Design review of the part built by this model. Coordinates are the model's own, in mm. Face numbers are marked on the shaded views. Coordinates: 2 decimals unless noted, no trailing zeros. Loops run counter-clockwise (first coordinate to the right, second up) from the corner with the lowest first, then second, coordinate; pieces in that order, holes last. Notation, with made-up numbers: (73, 87) - (94, 87) arc R16 cw to (94, 113) - close; hole circle Ø11 at (-4.75, -22). An arc over 180 degrees is marked (long way). One line per question, with ' | ' between items.
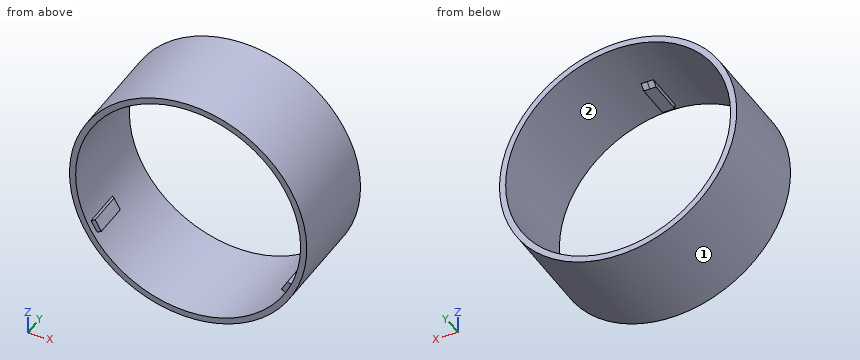
from build123d import *

# Parameters (mm, degrees)
SKETCH_1_R               = 38.5
SKETCH_1_R_2             = 36.5
EXTRUDE_1_DEPTH          = 40
EXTRUDE_3_DEPTH          = 1.6
PATTERN_CIRCULAR_1_COUNT = 3
SKETCH_3_R               = 52.927820275
CUT_EXTRUDE_1_DEPTH      = 7
CHAMFER_1_SIZE           = 1.7


with BuildPart() as part:
    # Эскиз1 → Бобышка-Вытянуть1 (new body)
    with BuildSketch(Plane(origin=(0, 0, 0), x_dir=(1, 0, 0), z_dir=(0, 1, 0))):
        with Locations(Location((0, 0, 0), (0, 0, 270))):
            Circle(SKETCH_1_R)
        with Locations(Location((0, 0, 0), (0, 0, 270))):
            Circle(SKETCH_1_R_2, mode=Mode.SUBTRACT)
    extrude(amount=EXTRUDE_1_DEPTH)

    # Эскиз2 → Бобышка-Вытянуть3 (add)
    with BuildSketch(Plane.XY.offset(36.5)):
        Polygon((1.95, 20.447072268), (-0.95, 20.447072268), (-2.05, 20.447072268), (-2.05, 9), (1.95, 9), align=None)
    extrude_3 = extrude(amount=-EXTRUDE_3_DEPTH)

    # Круговой массив1: Бобышка-Вытянуть3 ×3 about axis
    pattern_circular_1_axis = Axis((0, 0, 0), (0, 1, 0))
    for i in range(1, PATTERN_CIRCULAR_1_COUNT):
        add(extrude_3.rotate(pattern_circular_1_axis, i * 360 / PATTERN_CIRCULAR_1_COUNT))

    # Эскиз3 → Вырез-Вытянуть1 (cut)
    with BuildSketch(Plane.XZ):
        Circle(SKETCH_3_R)
    extrude(amount=-CUT_EXTRUDE_1_DEPTH, mode=Mode.SUBTRACT)

    # Фаска1
    # the kernel refuses this chamfer: 1.7 mm, written as the material it adds along each edge
    with BuildSketch(Plane(origin=(0, 20.447072268, 0), x_dir=(0, 0, 1), z_dir=(1, 0, 0))) as chamfer_1_piece_1_section:
        Polygon((36.5, -CHAMFER_1_SIZE), (36.5 - CHAMFER_1_SIZE, 0), (36.5, 0), align=None)
    chamfer_1_piece_1 = revolve(axis=Axis((0, 20.447072268, 0), (0, -1, 0)), revolution_arc=10.082397384, mode=Mode.PRIVATE)
    chamfer_1_piece_1 = split(chamfer_1_piece_1, bisect_by=Plane(origin=(-2.05, 21.014554038, 35.932884204), z_dir=(1, 0, 0)), keep=Keep.TOP, mode=Mode.PRIVATE)
    chamfer_1_piece_1 = split(chamfer_1_piece_1, bisect_by=Plane(origin=(-1.024016217, 21.014554038, 34.9), z_dir=(0, 0, 1)), keep=Keep.TOP, mode=Mode.PRIVATE)
    add(chamfer_1_piece_1)
    with BuildSketch(Plane(origin=(0, 20.447072268, 0), x_dir=(-0.9392452885856895, 0, -0.3432466866112253), z_dir=(-0.3432466866112253, 0, 0.9392452885856895))) as chamfer_1_piece_2_section:
        Polygon((36.5, -CHAMFER_1_SIZE), (36.5 - CHAMFER_1_SIZE, 0), (36.5, 0), align=None)
    chamfer_1_piece_2 = revolve(axis=Axis((0, 20.447072268, 0), (0, -1, 0)), revolution_arc=20.007603595, mode=Mode.PRIVATE)
    chamfer_1_piece_2 = split(chamfer_1_piece_2, bisect_by=Plane(origin=(-32.094466273, 21.014490137, -16.278082692), z_dir=(0.5000000000000004, 0, -0.8660254037844384)), keep=Keep.TOP, mode=Mode.PRIVATE)
    chamfer_1_piece_2 = split(chamfer_1_piece_2, bisect_by=Plane(origin=(-30.094466273, 21.014490137, -19.742184307), z_dir=(-0.5000000000000004, 0, 0.8660254037844384)), keep=Keep.TOP, mode=Mode.PRIVATE)
    chamfer_1_piece_2 = split(chamfer_1_piece_2, bisect_by=Plane(origin=(-30.199383778, 21.014490137, -17.493132939), z_dir=(-0.8660254037844384, 0, -0.5000000000000004)), keep=Keep.TOP, mode=Mode.PRIVATE)
    add(chamfer_1_piece_2)
    with BuildSketch(Plane(origin=(0, 20.447072268, 0), x_dir=(0.7668829946630015, 0, -0.6417869369944413), z_dir=(-0.6417869369944413, 0, -0.7668829946630015))) as chamfer_1_piece_3_section:
        Polygon((36.5, -CHAMFER_1_SIZE), (36.5 - CHAMFER_1_SIZE, 0), (36.5, 0), align=None)
    chamfer_1_piece_3 = revolve(axis=Axis((0, 20.447072268, 0), (0, -1, 0)), revolution_arc=20.007603595, mode=Mode.PRIVATE)
    chamfer_1_piece_3 = split(chamfer_1_piece_3, bisect_by=Plane(origin=(30.144466273, 21.014490137, -19.655581767), z_dir=(0.49999999999999983, 0, 0.8660254037844388)), keep=Keep.TOP, mode=Mode.PRIVATE)
    chamfer_1_piece_3 = split(chamfer_1_piece_3, bisect_by=Plane(origin=(32.144466273, 21.014490137, -16.191480152), z_dir=(-0.49999999999999983, 0, -0.8660254037844388)), keep=Keep.TOP, mode=Mode.PRIVATE)
    chamfer_1_piece_3 = split(chamfer_1_piece_3, bisect_by=Plane(origin=(30.249189406, 21.014490137, -17.406867061), z_dir=(0.8660254037844388, 0, -0.49999999999999983)), keep=Keep.TOP, mode=Mode.PRIVATE)
    add(chamfer_1_piece_3)
    with BuildSketch(Plane(origin=(0, 20.447072268, 0), x_dir=(0.17236211792697714, 0, 0.9850336544015776), z_dir=(0.9850336544015776, 0, -0.17236211792697714))) as chamfer_1_piece_4_section:
        Polygon((36.5, -CHAMFER_1_SIZE), (36.5 - CHAMFER_1_SIZE, 0), (36.5, 0), align=None)
    chamfer_1_piece_4 = revolve(axis=Axis((0, 20.447072268, 0), (0, -1, 0)), revolution_arc=9.925186074, mode=Mode.PRIVATE)
    chamfer_1_piece_4 = split(chamfer_1_piece_4, bisect_by=Plane(origin=(1.95, 21.014422977, 35.934484575), z_dir=(-1, 0, 0)), keep=Keep.TOP, mode=Mode.PRIVATE)
    chamfer_1_piece_4 = split(chamfer_1_piece_4, bisect_by=Plane(origin=(0.974165445, 21.014422977, 34.9), z_dir=(0, 0, 1)), keep=Keep.TOP, mode=Mode.PRIVATE)
    add(chamfer_1_piece_4)


solid = part.part
Q1. Take a section at B-B (x = 27.5). Give the boundary of the cut face in (y, z), plus the area to 3 significant figures.
Returned:
outline: (7, -26.94) - (40, -26.94) - (40, -24) - (7, -24) - close; (7, 24) - (40, 24) - (40, 26.94) - (7, 26.94) - close | area: 194 mm²
Q2. To check wall thickness, follow line 1 along Z through (x, y) = (0, 27); line 2 along Z through (x, y) = (-0.5, 10); line 3 along X through (y, z) = (25.5, 1). State the ranges of each line that lie inside material, in increasing order.
Returned:
line 1: z = -38.5 to -36.5, 36.5 to 38.5 | line 2: z = -38.5 to -36.5, 34.9 to 38.5 | line 3: x = -38.49 to -36.49, 36.49 to 38.49
Q3. For pin 1 (0.8 mm diameter, centred on x = 0.5, z = 36, fed in from -Y); pin 2 (4 mm diameter, centred on x = 4.5, y = 33.5, fed in from +Z); pin 3 (1 mm diameter, centred on y = 26.5, z = -10.5, fed in from -X); pin 4 (8 mm diameter, centred on x = 22, z = -26, fed in from +Y), all flat-tipped, find the tip position at first contact; note any pin that passes through.
Returned:
pin 1: stops at y = 9 | pin 2: stops at z = 38.42 | pin 3: stops at x = -37.18 | pin 4: stops at y = 40
Q4. Take a section at D-D (y = 25.5). Give the boundary of the cut face in (x, z), plus the area to 3 significant figures.
Returned:
outline: circle Ø77 at (0, 0); hole circle Ø73 at (0, 0) | area: 471 mm²
Q5. Take a section at C-C (y = 14). Give the boundary of the cut face in (x, z).
Returned:
outline: circle Ø77 at (0, 0); hole (-32.54, -16.54) - (-31.2, -15.76) - (-29.2, -19.23) - (-30.54, -20) arc R36.5 ccw to (30.59, -19.91) - (29.25, -19.14) - (31.25, -15.67) - (32.59, -16.45) arc R36.5 ccw to (1.95, 36.45) - (1.95, 34.9) - (-2.05, 34.9) - (-2.05, 36.44) arc R36.5 ccw to start
Q6. Take a section at A-A (z = 0). Give the boundary of the cut face in (x, y), plus the area to 3 significant figures.
Returned:
outline: (-38.5, 7) - (-36.5, 7) - (-36.5, 40) - (-38.5, 40) - close; (36.5, 7) - (38.5, 7) - (38.5, 40) - (36.5, 40) - close | area: 132 mm²
Q7. Draft analysis for pull direction X (two halves, no side actions). For the marked faces 1 and 2, state which applies: +X half, -X half, draft (parallel to the pull), parting line (faces both ways), or undercut.
Returned:
face 1: parting line | face 2: undercut
